Input: part model. Units: mm. Frame: model coordinates. A direction names the side the tool comes from. Round coordinates to 2 decimals unless told otherwise and drop trailing zeros. Loops run counter-clockwise (first coordinate to the right, second up) from the corner with the lowest first, then second, coordinate; pieces in that order, holes last. Notation, with made-up numbers: M 16,49 L 25,49 A32 ccw 25,79 Z; hole C 33,20 d4. An arc over 180 degrees is marked long. Use one line per item in the form item = value. Start each with the question number.
Q1. Mould query, pull axis Z, two halves, no side actions, for faces 1 (the flat face through (-79, -902, 88.306)), 2 (the flat face through (-117.254, -902, 51)), 3 (the flat face through (-80, -902, 13.375)). Classes: pulls with the +Z half, pulls with the -Z half, needs draft (parallel to the pull), parting line crosses it, or undercut.
Q2. Access query for faces 4 (the flat face through (-41.054, -902, 51)), 5 (the flat face through (-42.32, -902, 51)). Directions: +Z, -Z, +X, -X, +Y, -Y. A direction counts if a zero-diameter tool reaches every point of the face in a straight line with its end or side. Return the directions, or none.
Q3. Ray query, line 1 along Z through (x, y) = (-111, -891); line 2 along X through (y, z) = (-907.5, 73). Return the intervals inside material, ascending.
Q4. Section query B-B, the plane y = -898.25. Output: boundary loops of the cut face in (x, z).
Q5. Section query C-C, the plane x = -103. Output: boundary loops of the cut face in (y, z), and give its area (3 significant figures).
Q6. Section query A-A, the plane z = 41.5. Output: boundary loops of the cut face in (x, y).
```python
from build123d import *

# Parameters (mm, degrees)
F0_W     = 76.2
F0_H     = 76.2
F1_DEPTH = 609.6
F3_DEPTH = 914.4
F4_DEPTH = 304.8
F5_DEPTH = 508
F6_DEPTH = 381


with BuildPart() as f1:
    # F0 (on Front) → F1 (new body)
    with BuildSketch(Plane.XZ):
        with Locations((-79.1539917648, 51.4746750653)):
            Rectangle(F0_W, F0_H)
    extrude(amount=F1_DEPTH)

    # F2 (on face) → F3 (cut)
    with BuildSketch(Plane.XZ.offset(609.6)):
        Polygon((-42.3204526305, 88.3055701852), (-98.6881405115, 88.3055701852), (-115.9909814596, 88.3055701852), (-115.9909814596, 14.655277133), (-42.3204526305, 14.655277133), align=None)
    extrude(amount=-F3_DEPTH, mode=Mode.SUBTRACT)

    # F4 (add): a face of the model
    f4_faces = [f1.faces().sort_by_distance(p)[0] for p in [
        (-42.1316224993, -609.6, 51.4746750653),
    ]]
    extrude(f4_faces, amount=F4_DEPTH)

    # F5 (cut): a face of the model
    f5_faces = [f1.faces().sort_by_distance(p)[0] for p in [
        (-42.1316224993, 0, 51.4746750653),
    ]]
    extrude(f5_faces, amount=-F5_DEPTH, mode=Mode.SUBTRACT)

    # F6 (cut): a face of the model
    f6_faces = [f1.faces().sort_by_distance(p)[0] for p in [
        (-42.1316224993, -508, 51.4746750653),
    ]]
    extrude(f6_faces, amount=-F6_DEPTH, mode=Mode.SUBTRACT)


solid = f1.part
```
Results found:
q1.face_1 = undercut
q1.face_2 = needs draft
q1.face_3 = pulls with the -Z half
q2.face_4 = +Z, -Z, +X, +Y, -Y
q2.face_5 = +Y, -Y
q3.line_1 = 13.37 to 14.66, 88.31 to 89.57
q3.line_2 = -117.25 to -115.99, -42.32 to -41.05
q4.outline = M -117.25,13.37 L -41.05,13.37 L -41.05,89.57 L -117.25,89.57 Z; hole M -115.99,14.66 L -42.32,14.66 L -42.32,88.31 L -115.99,88.31 Z
q5.outline = M -914.4,13.37 L -889,13.37 L -889,14.66 L -914.4,14.66 Z; M -914.4,88.31 L -889,88.31 L -889,89.57 L -914.4,89.57 Z
q5.area = 64.8 mm²
q6.outline = M -117.25,-914.4 L -115.99,-914.4 L -115.99,-889 L -117.25,-889 Z; M -42.32,-914.4 L -41.05,-914.4 L -41.05,-889 L -42.32,-889 Z
